Read the model definition and answer for the solid it produces. Units are mm, in the model's axes. A direction names the side the tool comes from. Round coordinates to 2 decimals unless told otherwise and drop trailing zeros. Order: outer loops, then holes, each group sorted by start corner. A loop starts at its lowest first (then second) coordinate and runs counter-clockwise, first axis right, second up. Notation, with made-up numbers: (-38.5, 26.5) -> (-6.5, 26.5) arc R27 cw to (-6.5, 47.5) -> close; hole circle Ø7 at (-15.75, 62). An arc over 180 degrees is marked (long way). Answer as a JSON object with one key per item and string values. Group by question number.
Item 1: Section B-B, the plane x = 50.5 is taken. Write down the section's boundary in (y, z) (3 decimals), plus the area to 4 significant figures.
Item 2: Section C-C, the plane y = 6 is taken. Write down the section's boundary in (x, z).
Item 3: For faces 1 (the flat face through (-52, 3, 5)), 2 (the flat face through (42, 0, 9)), 3 (the flat face through (-1, 0, 0)), 4 (the flat face through (-1, 0, 5)), 5 (the flat face through (49, 3, 5)), determine the directions among +Z, -Z, +X, -X, +Y, -Y from which every point of the face is accessible in a straight line to the end or side of a thin tool.
Item 4: Section A-A, the plane y = 0 is taken. Write down the section's boundary in (x, z) (3 decimals), plus the area to 4 significant figures.
Item 5: Section D-D, the plane z = 2.5 is taken. Write down the section's boundary in (x, y) (3 decimals).
Item 6: Consider probe 1 along Y at (x, z) = (-41.5, 6.5); probe 2 along Y at (x, z) = (50.5, 4) (3 decimals); probe 3 along Z at (x, y) = (50, -3). Determine where each line is inside the solid, lowest interval first. Write a range as from..to.
Item 7: Given P1, Ø4, axis at y = -4.5, z = 8, coming from the +X side; P2, Ø7.5, axis at x = -52, y = -5.5, coming from the +Z side, each flat-ended and moving along its own axis, determine where each tip first touches the part or whether it passes through.
Item 8: The mould has two halves that part along X. Classify faces 6 (the flat face through (-40, -0.2, 5.8)), 7 (the flat face through (40, 0.2, 5.8)), 8 (the flat face through (-41, 0, 9)), 9 (the flat face through (-43, 0.2, 5.8)): pulls with the +X half, pulls with the -X half, needs draft (parallel to the pull), parting line crosses it, or undercut.
Autodesk Fusion 360 part; units mm, degrees
sketch "Sketch1" plane through (0, 0, 0) normal (0, 0, 1) x (1, 0, 0)
  line L0 (40, -11) -> (-40, -11)
  line L1 (-40, -11) -> (-40, 11)
  line L2 (-40, 11) -> (40, 11)
  line L3 (40, 11) -> (40, -11)
  line L4 (40, -11) -> (-40, 11) construction
  line L5 (-40, -11) -> (40, 11) construction
  line L6 (-40, 11) -> (-43, 11)
  line L7 (-43, 11) -> (-43, -11)
  line L8 (-43, -11) -> (-40, -11)
  line L9 (-40, -11) -> (-40, 11)
  line L10 (40, 11) -> (43, 11)
  line L11 (43, 11) -> (43, -11)
  line L12 (43, -11) -> (40, -11)
  line L13 (40, -11) -> (40, 11)
  line L14 (43, 11) -> (58, 11)
  line L15 (58, 11) -> (58, -11)
  line L16 (58, -11) -> (43, -11)
  line L17 (43, -11) -> (43, 11)
  line L18 (-43, 11) -> (-58, 11)
  line L19 (-58, 11) -> (-58, -11)
  line L20 (-58, -11) -> (-43, -11)
  line L21 (-43, -11) -> (-43, 11)
  circle A0 centre (-50.5, 0) radius 2.625
  circle A1 centre (50.5, 0) radius 2.625
  dimension "d1" = 80
  dimension "d2" = 22
  dimension "d3" = 3
  dimension "d4" = 22
  dimension "d5" = 3
  dimension "d6" = 15
  dimension "d7" = 22
  dimension "d8" = 15
  dimension "d9" = 22
  dimension "d10" = 5.25
  dimension "d11" = 5.25
  dimension "d19" = 22
extrude "Extrude1" add sketch "Sketch1" along normal blind 5 contours L0 L1 L2 L3 L9 L13 | L11 L14 L15 L16 L17 | L7 L18 L19 L20 L21 makes body 1 at (50.5654, -8.2059, 0) makes body 2 at (13.3333, -3.6667, 0) makes body 3 at (-50.4346, -8.2059, 0)
extrude "Extrude2" add sketch "Sketch1" along normal blind 10 contours L3 L10 L11 L12 L13 L17 | L1 L6 L7 L8 L9 L21 bodies 1 2 3
sketch "Sketch2" plane through (43, 0, 0) normal (1, 0, 0) x (0, 1, 0)
  line L0 (-11, 5) -> (11, 5)
  line L1 (11, 5) -> (11, 10)
  line L2 (11, 10) -> (-11, 10)
  line L3 (-11, 10) -> (-11, 5)
  line L4 (-11, 10) -> (11, 10)
  line L5 (11, 10) -> (11, 5)
  line L6 (11, 5) -> (-11, 5)
  line L7 (-11, 5) -> (-11, 10)
  line L8 (10, 6) -> (-10, 6)
  line L9 (-10, 6) -> (-10, 9)
  line L10 (-10, 9) -> (10, 9)
  line L11 (10, 9) -> (10, 6)
  dimension "d16" = 1
extrude "Extrude3" cut sketch "Sketch2" against normal up to surface (86 mm away) contours L8 L9 L10 L11 bodies 1
equation "d4 = d2"
equation "d7 = d2"
equation "d9 = d2"
equation "d19 = d2"
Values found:
{
 "1": {"outline": "(-11, 0) -> (-2.625, 0) -> (-2.625, 5) -> (-11, 5) -> close; (2.625, 0) -> (11, 0) -> (11, 5) -> (2.625, 5) -> close", "area": "83.75 mm2"},
 "2": {"outline": "(-58, 0) -> (58, 0) -> (58, 5) -> (43, 5) -> (43, 6) -> (40, 6) -> (40, 5) -> (-40, 5) -> (-40, 6) -> (-43, 6) -> (-43, 5) -> (-58, 5) -> close; (-43, 9) -> (-40, 9) -> (-40, 10) -> (-43, 10) -> close; (40, 9) -> (43, 9) -> (43, 10) -> (40, 10) -> close"},
 "3": {"face 1": "+Z, -X, +Y, -Y", "face 2": "+X, -X", "face 3": "-Z, +X, -X, +Y, -Y", "face 4": "+Z, +Y, -Y", "face 5": "+Z, +X, +Y, -Y"},
 "4": {"outline": "(-58, 0) -> (-53.125, 0) -> (-53.125, 5) -> (-58, 5) -> close; (-47.875, 0) -> (47.875, 0) -> (47.875, 5) -> (43, 5) -> (43, 6) -> (40, 6) -> (40, 5) -> (-40, 5) -> (-40, 6) -> (-43, 6) -> (-43, 5) -> (-47.875, 5) -> close; (-43, 9) -> (-40, 9) -> (-40, 10) -> (-43, 10) -> close; (40, 9) -> (43, 9) -> (43, 10) -> (40, 10) -> close; (53.125, 0) -> (58, 0) -> (58, 5) -> (53.125, 5) -> close", "area": "539.5 mm2"},
 "5": {"outline": "(-58, -11) -> (58, -11) -> (58, 11) -> (-58, 11) -> close; hole circle Ø5.25 at (-50.5, 0); hole circle Ø5.25 at (50.5, 0)"},
 "6": {"probe 1": "-11..-10, 10..11", "probe 2": "-11..-2.625, 2.625..11", "probe 3": "0..5"},
 "7": {"P1": "x = 43", "P2": "z = 5"},
 "8": {"face 6": "undercut", "face 7": "undercut", "face 8": "needs draft", "face 9": "pulls with the -X half"}
}
